Could you check a few things on this drawing? It's one solid part, dimensions in mm from its lowest x, y, z. A direction names the side the tool comes from. Coordinates: 2 decimals unless noted, no trailing zeros. Order: outer loops, then holes, each group sorted by start corner. A loop starts at its lowest first (then second) coordinate and runs counter-clockwise, first axis right, second up.
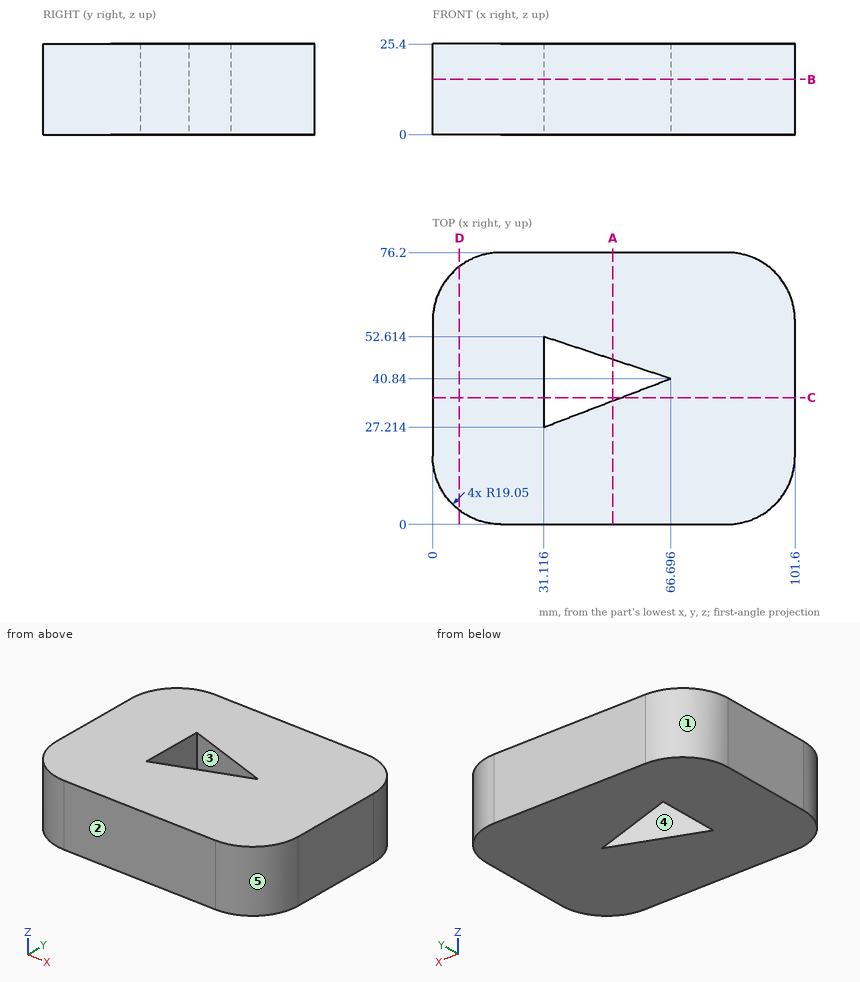
1. Imagine slicing it at A-A on x = 50.5. Please give me the cut outline in (y, z).
Completed:
outline: (0, 0) - (34.64, 0) - (34.64, 25.4) - (0, 25.4) - close; (46.2, 0) - (76.2, 0) - (76.2, 25.4) - (46.2, 25.4) - close
2. I'm going to push a flat-ended pin straight in: pin 1 (8 mm diameter, centred on x = 90, z = 13, fed in from +Y) (1 decimal). Where does the tip first touch, or does it pass through?
Completed:
pin 1: stops at y = 75.9
3. On a 3-axis mill with a long thin cutter (end or side, diameter ignored), from which of +Z, -Z, +X, -X, +Y, -Y can I reach the whole of each face in a straight line? I mean the marked faces 4 and 5. Say none if no direction works.
Completed:
face 4: +Z, -Z
face 5: +Z, -Z, +X, -Y
4. Thinking about a two-plate mould opening in Y: for the marked faces 1, 2 and 3, which applies, pulls with the +Y half, pulls with the -Y half, needs draft (parallel to the pull), parting line crosses it, or undercut?
Completed:
face 1: pulls with the +Y half
face 2: pulls with the -Y half
face 3: undercut
5. Imagine slicing it at D-D on x = 7.5. Please give me the cut outline in (y, z), then the cut area to 3 significant figures.
Completed:
outline: (3.9, 0) - (72.3, 0) - (72.3, 25.4) - (3.9, 25.4) - close
area: 1,740 mm2
6. Please list where these lines run through material, in increasing order: probe 1 along Y at (x, z) = (83, 16.75) (1 decimal); probe 2 along Y at (x, z) = (56.5, 7) (1 decimal); probe 3 along Y at (x, z) = (32, 20.5).
Completed:
probe 1: y = 0 to 76.2
probe 2: y = 0 to 36.9, 44.2 to 76.2
probe 3: y = 0 to 27.55, 52.32 to 76.2
7. Imagine slicing it at C-C on y = 35.5. Please give me the cut outline in (x, z).
Completed:
outline: (0, 0) - (31.12, 0) - (31.12, 25.4) - (0, 25.4) - close; (52.75, 0) - (101.6, 0) - (101.6, 25.4) - (52.75, 25.4) - close
8. Imagine slicing it at B-B on z = 15.5. Please give me the cut outline in (x, y), then the cut area to 3 significant figures.
Completed:
outline: (0, 19.05) arc R19.05 ccw to (19.05, 0) - (82.55, 0) arc R19.05 ccw to (101.6, 19.05) - (101.6, 57.15) arc R19.05 ccw to (82.55, 76.2) - (19.05, 76.2) arc R19.05 ccw to (0, 57.15) - close; hole (31.12, 27.21) - (66.7, 40.84) - (31.12, 52.61) - close
area: 6,980 mm2
